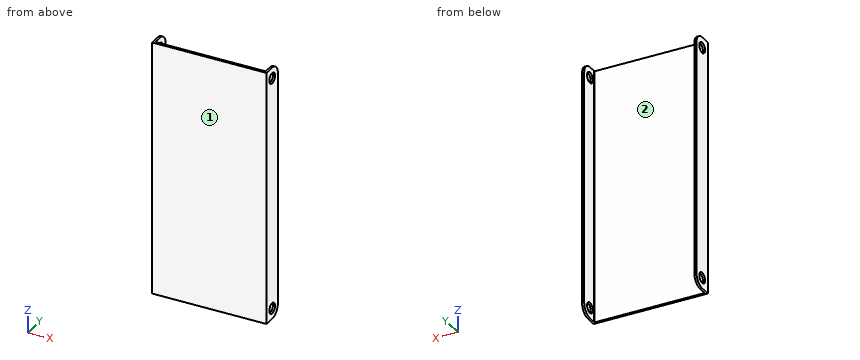
from build123d import *

# Parameters (mm, degrees)
BOSS_EXTRUDE1_DEPTH = 152.4
SKETCH2_R           = 3.175
CUT_EXTRUDE1_DEPTH  = 69.58
FILLET1_R           = 0.635


with BuildPart() as part:
    # Sketch1 → Boss-Extrude1 (new body)
    with BuildSketch(Plane.XY):
        Polygon((-34.29, 6.35), (-34.29, -6.35), (34.29, -6.35), (34.29, 6.35), (33.02, 6.35), (33.02, -5.08), (-33.02, -5.08), (-33.02, 6.35), align=None)
    extrude(amount=BOSS_EXTRUDE1_DEPTH)

    # Sketch2 → Cut-Extrude1 (cut, through all)
    with BuildSketch(Plane(origin=(34.29, 0, 0), x_dir=(0, 0, -1), z_dir=(1, 0, 0))):
        with Locations((-146.05, 0)):
            Circle(SKETCH2_R)
        with Locations((-6.35, 0)):
            Circle(SKETCH2_R)
        with BuildLine():
            Line((-152.4, 0), (-152.4, 6.35))
            Line((-152.4, 6.35), (-146.05, 6.35))
            ThreePointArc((-146.05, 6.35), (-150.540128061, 4.490128061), (-152.4, 0))
        make_face()
        with BuildLine():
            Line((0, 0), (0, 6.35))
            Line((0, 6.35), (-6.35, 6.35))
            ThreePointArc((-6.35, 6.35), (-1.859871939, 4.490128061), (0, 0))
        make_face()
    extrude(amount=-CUT_EXTRUDE1_DEPTH, mode=Mode.SUBTRACT)

    # Fillet1
    fillet1_edges = [part.edges().sort_by_distance(p)[0] for p in [
        (-33.02, -5.08, 76.2),
        (33.02, -5.08, 76.2),
    ]]
    fillet(fillet1_edges, radius=FILLET1_R)


solid = part.part
Could you check a few things on this model? Use its own coordinates, in mm. Face numbers are marked on the shaded views. Round coordinates to 2 decimals unless told otherwise and drop trailing zeros. Order: outer loops, then holes, each group sorted by start corner. A loop starts at its lowest first (then second) coordinate and runs counter-clockwise, first axis right, second up.
(1) Imagine slicing it at A-A (y = 1.5). Write out the boundary of the cut face in (x, z), plus the area to 3 significant figures.
Response values:
outline: (-34.29, 0.18) - (-33.02, 0.18) - (-33.02, 3.55) - (-34.29, 3.55) - close; (-34.29, 9.15) - (-33.02, 9.15) - (-33.02, 143.25) - (-34.29, 143.25) - close; (-34.29, 148.85) - (-33.02, 148.85) - (-33.02, 152.22) - (-34.29, 152.22) - close; (33.02, 0.18) - (34.29, 0.18) - (34.29, 3.55) - (33.02, 3.55) - close; (33.02, 9.15) - (34.29, 9.15) - (34.29, 143.25) - (33.02, 143.25) - close; (33.02, 148.85) - (34.29, 148.85) - (34.29, 152.22) - (33.02, 152.22) - close
area: 358 mm2
(2) I'm going to push a flat-ended pin straight in: pin 1 (8 mm diameter, centred on x = 16.5, z = 103, fed in from +Y). Where does the tip first touch, or does it pass through?
Response values:
pin 1: stops at y = -5.08
(3) If we mould it in two halves opening along X, with no side actions, what happens to the marked faces 1 and 2? For each: released by +X, released by -X, zero draft, split by the parting line, or undercut.
Response values:
face 1: zero draft
face 2: undercut
(4) Please list where these lines run through material, in increasing order: line 1 along X through (y, z) = (2.5, 106); line 2 along Y through (x, z) = (33.8, 146.05) (3 decimals).
Response values:
line 1: x = -34.29 to -33.02, 33.02 to 34.29
line 2: y = -6.35 to -3.175, 3.175 to 6.35
(5) Imagine slicing it at B-B (z = 110). Write out the boundary of the cut face in (x, y) (3 decimals), plus the area to 3 significant figures.
Response values:
outline: (-34.29, -6.35) - (34.29, -6.35) - (34.29, 6.35) - (33.02, 6.35) - (33.02, -4.445) arc R0.635 cw to (32.385, -5.08) - (-32.385, -5.08) arc R0.635 cw to (-33.02, -4.445) - (-33.02, 6.35) - (-34.29, 6.35) - close
area: 116 mm2
(6) Imagine slicing it at C-C (x = 4). Write out the boundary of the cut face in (y, z), plus the area to 3 significant figures.
Response values:
outline: (-6.35, 0) - (-5.08, 0) - (-5.08, 152.4) - (-6.35, 152.4) - close
area: 194 mm2
